Can you work these out from the model? Positions are in its coordinate system, mm. Give positions to 0.01 mm unless a question says otherwise; leave off trailing zeros. Order: outer loops, then holes, each group sorted by start corner. A loop starts at its lowest first (then second) coordinate and runs counter-clockwise, first axis right, second up. Notation, with made-up numbers: (-20.75, -26.75) - (31.25, -26.75) arc R5 cw to (31.25, -22.75) - close; hole circle Ø3 at (58, 73). An arc over 180 degrees is marked (long way). Return JSON: item names as keys, results as strings.
Autodesk Inventor part; units mm, degrees
ref_plane "YZ Plane" through (0, 0, 0) normal (1, 0, 0) x (0, 1, 0)
ref_plane "XZ Plane" through (0, 0, 0) normal (0, 1, 0) x (-1, 0, 0)
ref_plane "XY Plane" through (0, 0, 0) normal (0, 0, 1) x (1, 0, 0)
sketch "Sketch1" plane through (0, 0, 0) normal (0, 1, 0) x (-1, 0, 0)
  line L0 (0, 0) -> (0, -10)
  line L1 (0, -10) -> (20, -10)
  line L2 (20, -10) -> (20, 0)
  line L3 (20, 0) -> (0, 0)
  line L4 (0, -5) -> (5, -5)
  circle A0 centre (5, -5) radius 2.6
  dimension "d0" = 10
  dimension "d1" = 20
  dimension "d2" = 5
  dimension "d3" = 5.2
extrude "Extrusion1" add sketch "Sketch1" along normal blind 10
sketch "Sketch2" plane through (-20, 0, 0) normal (0, 0, 1) x (1, 0, 0)
  line L0 (0, 10) -> (0, 0)
  line L1 (0, 0) -> (0, 10)
  line L2 (0, 5) -> (5, 5)
  circle A0 centre (5, 5) radius 2.6
  point P0 (20, 0)
  dimension "d6" = 5
  dimension "d7" = 5.2
extrude "Extrusion2" cut sketch "Sketch2" against normal blind 11
properties part number "roller_joint"
1. Suppose I cut it at B-B (y = 5). List the corners of the cut face in (x, z) for me, plus the area to 3 significant figures.
Checks:
{"outline": "(-20, -10) - (-17.6, -10) - (-17.6, 0) - (-20, 0) - close; (-12.4, -10) - (0, -10) - (0, 0) - (-12.4, 0) - close; hole circle Ø5.2 at (-5, -5)", "area": "127 mm^2"}
2. Thinking about a two-plate mould opening in Z: for faces 1 (the face through (-4.662, 4.93, -7.578)), 2 (the face through (-10, 10, -5)), 3 (the face through (-10, 5, 0)), which applies, +Z half, -Z half, draft (parallel to the pull), parting line (faces both ways), or undercut?
Checks:
{"face 1": "undercut", "face 2": "draft", "face 3": "+Z half"}
3. Suppose I cut it at D-D (y = 9). List the corners of the cut face in (x, z) for me.
Checks:
{"outline": "(-20, -10) - (0, -10) - (0, 0) - (-20, 0) - close; hole circle Ø5.2 at (-5, -5)"}
4. If I drill on L1, parallel to X at y = 6.5, z = -7; L2, parallel to Y at x = -15, z = -0.75; L3, parallel to X at y = 3.5, z = -4, over which ranges is the centre line in solid material (lowest first)? Write a range as [from, to].
Checks:
{"L1": "[-20, -17.12], [-12.88, -6.66], [-3.34, 0]", "L2": "[0, 2.4], [7.6, 10]", "L3": "[-20, -17.12], [-12.88, -7.4], [-2.6, 0]"}
5. Suppose I cut it at A-A (z = -5). List the corners of the cut face in (x, y) for me, plus the area to 3 significant figures.
Checks:
{"outline": "(-20, 0) - (-7.6, 0) - (-7.6, 10) - (-20, 10) - close; (-2.4, 0) - (0, 0) - (0, 10) - (-2.4, 10) - close; hole circle Ø5.2 at (-15, 5)", "area": "127 mm^2"}
6. Suppose I cut it at C-C (x = -5). List the corners of the cut face in (y, z) for me, plus the area to 3 significant figures.
Checks:
{"outline": "(0, -10) - (10, -10) - (10, -7.6) - (0, -7.6) - close; (0, -2.4) - (10, -2.4) - (10, 0) - (0, 0) - close", "area": "48.0 mm^2"}
